Verification items for the finished model (mm, model axes). A direction names the side the tool comes from. Give positions to 0.01 mm unless a question says otherwise; leave off trailing zeros. Write each loop counter-clockwise with the first axis right and the second up, starting at its lowest first coordinate (ties: lowest second). Pieces come first, ordered by that corner, then holes. Notation, with made-up numbers: (69, -7) -> (93, -7) arc R21 ccw to (93, 5) -> close; hole circle Ø10 at (-31.5, -8.75). An arc over 180 degrees is marked (long way). Write item = value, one per line.
Autodesk Inventor part; units mm, degrees
ref_plane "YZ Plane" through (0, 0, 0) normal (1, 0, 0) x (0, 1, 0)
ref_plane "XZ Plane" through (0, 0, 0) normal (0, 1, 0) x (-1, 0, 0)
ref_plane "XY Plane" through (0, 0, 0) normal (0, 0, 1) x (1, 0, 0)
sketch "Sketch1" plane through (0, 0, 0) normal (0, 1, 0) x (-1, 0, 0)
  line L0 (0, 0) -> (100, 0)
  line L1 (100, 0) -> (100, -178)
  line L2 (0, -178) -> (0, 0)
  line L3 (90, -10) -> (10, -10)
  line L4 (90, -52) -> (10, -52)
  line L5 (90, -62) -> (10, -62)
  line L6 (90, -52) -> (90, -10)
  line L7 (10, -10) -> (10, -52)
  line L8 (90, -118) -> (10, -118)
  line L9 (90, -168) -> (90, -128)
  line L10 (90, -118) -> (90, -62)
  line L11 (10, -62) -> (10, -118)
  line L12 (10, -128) -> (10, -168)
  line L13 (100, -178) -> (90, -178)
  line L14 (10, -178) -> (0, -178)
  line L15 (90, -168) -> (90, -178)
  line L16 (10, -168) -> (46, -168)
  line L17 (56, -168) -> (56, -178)
  line L18 (56, -178) -> (10, -178)
  line L19 (56, -168) -> (56, -128)
  line L20 (46, -128) -> (46, -168)
  line L21 (90, -128) -> (56, -128)
  line L22 (46, -128) -> (10, -128)
  dimension "thickness" = 10
  dimension "d3" = 10
  dimension "d4" = 10
  dimension "d8" = 10
  dimension "motor" = 42
  dimension "d10" = 10
  dimension "d11" = 10
  dimension "d27" = 10
  dimension "batterywidth" = 56
  dimension "d31" = 80
  dimension "suspensionWidth" = 40
  dimension "d33" = 10
  dimension "d34" = 10
  dimension "suspensionHeight" = 34
  dimension "d36" = 10
  dimension "d38" = 10
  dimension "d39" = 40
  dimension "d40" = 40
  dimension "d41" = 36
extrude "Extrusion2" add sketch "Sketch1" along normal blind 10
sketch "Sketch2" plane through (0, 10, 0) normal (0, 1, 0) x (1, 0, 0)
  line L0 (-100, 0) -> (-90, 0)
  line L1 (-90, 0) -> (-90, 10)
  line L2 (-90, 10) -> (-100, 10)
  line L3 (-100, 10) -> (-100, 0)
  line L4 (-10, 52) -> (-10, 10)
  line L5 (0, 0) -> (-10, 0)
  line L6 (-10, 0) -> (-10, 10)
  line L7 (-10, 10) -> (0, 10)
  line L8 (0, 10) -> (0, 0)
  line L9 (-100, 178) -> (-100, 0)
  line L10 (-100, 0) -> (0, 0)
  line L11 (-100, 52) -> (-90, 52)
  line L12 (-90, 52) -> (-90, 62)
  line L13 (-90, 62) -> (-100, 62)
  line L14 (-100, 62) -> (-100, 52)
  line L15 (-90, 52) -> (-10, 52)
  line L16 (-10, 52) -> (0, 52)
  line L17 (0, 52) -> (0, 62)
  line L18 (0, 62) -> (-10, 62)
  line L19 (-10, 62) -> (-10, 52)
  line L20 (-90, 10) -> (-90, 52)
  line L21 (-100, 118) -> (-90, 118)
  line L22 (-90, 118) -> (-90, 128)
  line L23 (-90, 128) -> (-100, 128)
  line L24 (-100, 128) -> (-100, 118)
  line L25 (-56, 128) -> (-90, 128)
  line L26 (-56, 118) -> (-46, 118)
  line L27 (-46, 118) -> (-46, 128)
  line L28 (-46, 128) -> (-56, 128)
  line L29 (-56, 128) -> (-56, 118)
  line L30 (-90, 118) -> (-10, 118)
  line L31 (0, 178) -> (-56, 178)
  line L32 (-10, 168) -> (0, 168)
  line L33 (0, 168) -> (0, 178)
  line L34 (0, 178) -> (-10, 178)
  line L35 (-10, 178) -> (-10, 168)
  line L36 (0, 0) -> (0, 178)
  line L37 (-10, 118) -> (0, 118)
  line L38 (0, 118) -> (0, 128)
  line L39 (0, 128) -> (-10, 128)
  line L40 (-10, 128) -> (-10, 118)
  line L41 (-10, 128) -> (-46, 128)
  line L42 (-56, 158) -> (-46, 158)
  line L43 (-46, 158) -> (-46, 168)
  line L44 (-46, 168) -> (-56, 168)
  line L45 (-56, 168) -> (-56, 158)
  line L46 (-46, 168) -> (-10, 168)
  line L47 (-46, 128) -> (-46, 168)
  line L48 (-100, 158) -> (-90, 158)
  line L49 (-90, 158) -> (-90, 168)
  line L50 (-90, 168) -> (-100, 168)
  line L51 (-100, 168) -> (-100, 158)
  line L52 (-90, 128) -> (-90, 178)
  dimension "d36" = 10
  dimension "d44" = 10
  dimension "d45" = 10
  dimension "d47" = 10
  dimension "d50" = 10
  dimension "d51" = 10
  dimension "d52" = 10
  dimension "d53" = 10
  dimension "d58" = 10
  dimension "d64" = 10
  dimension "d65" = 10
  dimension "d148" = 10
  dimension "d149" = 10
  dimension "d150" = 10
  dimension "d151" = 10
extrude "Extrusion3" add sketch "Sketch2" along normal blind 10 contours L3 L2 L1 L0 | L6 L7 L8 L5 | L9 L13 L12 L11 | L19 L18 L17 L16 | L9 L23 L22 L21 | L9 L50 L49 L48 | L29 L28 L27 L26 | L37 L40 L39 L36 | L32 L35 L31 L33 | L42 L45 L44 L43
sketch "Sketch6" plane through (0, 0, 0) normal (0, -1, 0) x (1, 0, 0)
  line L0 (-90, -10) -> (-80, -10)
  line L1 (-80, -10) -> (-80, -52)
  line L2 (-80, -52) -> (-90, -52)
  line L3 (-90, -52) -> (-90, -10)
  line L4 (-90, -52) -> (-90, -10)
  line L5 (-90, -10) -> (-10, -10)
  line L6 (-10, -52) -> (-90, -52)
  line L7 (-20, -10) -> (-10, -10)
  line L8 (-10, -10) -> (-10, -52)
  line L9 (-10, -52) -> (-20, -52)
  line L10 (-20, -52) -> (-20, -10)
  line L11 (-10, -10) -> (-10, -52)
  point P0 (0, 0)
  dimension "motorFixtureHeight" = 60
  dimension "d72" = 10
extrude "Extrusion5" add sketch "Sketch6" against normal blind 10 contours L0 L1 L2 L3 | L5 L8 L6 L10
sketch "Sketch7" plane through (0, 10, 0) normal (0, 1, 0) x (1, 0, 0)
  line L0 (-80, 10) -> (-20, 10)
  line L1 (-20, 10) -> (-20, 52)
  line L2 (-20, 52) -> (-80, 52)
  line L3 (-80, 52) -> (-80, 10)
  line L4 (-80, 10) -> (-80, 52)
  line L5 (-80, 52) -> (-20, 52)
  line L6 (-20, 52) -> (-20, 10)
  line L7 (-20, 10) -> (-80, 10)
  circle A0 centre (-50, 31) radius 18.75
  circle A1 centre (-75, 16) radius 2.1
  circle A2 centre (-25, 31) radius 2.1
  circle A3 centre (-75, 46) radius 2.1
  circle A4 centre (-25, 16) radius 2.1
  circle A5 centre (-25, 46) radius 2.1
  circle A6 centre (-75, 31) radius 2.1
  point P0 (0, 0)
  dimension "d75" = 37.5
  dimension "d77" = 21
  dimension "d78" = 30
  dimension "d79" = 4.2
  dimension "d80" = 4.2
  dimension "d82" = 4.2
  dimension "d83" = 4.2
  dimension "d84" = 4.2
  dimension "d85" = 4.2
  dimension "d86" = 25
  dimension "d87" = 0
  dimension "d88" = 25
  dimension "d89" = 15
  dimension "d90" = 25
  dimension "d91" = 15
  dimension "d92" = 15
  dimension "d93" = 25
  dimension "d94" = 25
  dimension "d95" = 0
  dimension "d96" = 25
  dimension "d97" = 15
extrude "Extrusion6" add sketch "Sketch7" against normal blind 6
hole "Hole2" at (0, 15, -173) direction (-1, 0, 0) diameter 4.3 end through all
hole "Hole3" at (0, 15, -123) direction (-1, 0, 0) diameter 4.3 end through all
hole "Hole4" at (0, 15, -57) direction (-1, 0, 0) diameter 4.3 end through all
hole "Hole5" at (0, 15, -5) direction (-1, 0, 0) diameter 4.3 end through all
sketch "Sketch8" plane through (-100, 0, -178) normal (-1, 0, 0) x (0, 0, 1)
  line L0 (116, 10) -> (60, 10)
  line L1 (60, 10) -> (60, 7)
  line L2 (60, 7) -> (116, 7)
  line L3 (116, 7) -> (116, 10)
  line L4 (116, 10) -> (60, 7) construction
  line L5 (60, 10) -> (116, 7) construction
  line L6 (60, 10) -> (116, 10)
  line L7 (60, 10) -> (60, 20)
  line L8 (116, 10) -> (116, 20)
  point P0 (178, 0)
  point P1 (88, 8.5)
  dimension "d145" = 3
extrude "Extrusion7" cut sketch "Sketch8" against normal up to surface (100 mm away)
hole "Hole6" at (-95, 15, -168) direction (0, 0, 1) diameter 4.3 depth 10 tip angle 118
hole "Hole7" at (-51, 15, -168) direction (0, 0, 1) diameter 4.3 depth 10 tip angle 118
sketch "Sketch9" plane through (-56, 0, -128) normal (0, 0, -1) x (-1, 0, 0)
  circle A0 centre (27, 5) radius 3.1
  circle A1 centre (7, 5) radius 3.1
  line L0 (34, 0) -> (0, 0)
  line L1 (0, 0) -> (0, 10)
  line L2 (34, 0) -> (34, 10)
  point P0 (-56, 0)
  dimension "d170" = 6.2
  dimension "d171" = 6.2
  dimension "d172" = 5
  dimension "d173" = 5
  dimension "d174" = 7
  dimension "d175" = 7
extrude "Extrusion8" cut sketch "Sketch9" against normal blind 5
equation "\"d3\" = thickness"
equation "\"d4\" = thickness"
equation "\"d8\" = thickness"
equation "\"d10\" = thickness"
equation "\"d11\" = thickness"
equation "\"d27\" = thickness"
equation "\"d33\" = thickness"
equation "\"d34\" = thickness"
equation "\"d36\" = thickness"
equation "\"d38\" = thickness"
equation "\"d39\" = suspensionWidth"
equation "\"d40\" = suspensionWidth"
equation "\"d42\" = thickness"
equation "\"d44\" = thickness"
equation "\"d50\" = thickness"
equation "\"d51\" = thickness"
equation "\"d52\" = thickness"
equation "\"d53\" = thickness"
equation "\"d58\" = thickness"
equation "\"d64\" = thickness"
equation "\"d65\" = thickness"
equation "\"d148\" = thickness"
equation "\"d149\" = thickness"
equation "\"d150\" = thickness"
equation "\"d151\" = thickness"
equation "\"d66\" = thickness"
equation "\"d73\" = thickness"
equation "\"d77\" = 0.5 * motor"
equation "\"d159\" = thickness"
equation "\"d168\" = thickness"
properties part number "sideFrame" material "ABS Plastic"
Item 1: Sectioned sample at B-B on z = -31. Record the cut outline in (x, y), then the cut area to 3 significant figures.
Response values:
outline = (-100, 0) -> (-80, 0) -> (-80, 4) -> (-77.1, 4) -> (-77.1, 10) -> (-100, 10) -> close; (-72.9, 4) -> (-68.75, 4) -> (-68.75, 10) -> (-72.9, 10) -> close; (-31.25, 4) -> (-27.1, 4) -> (-27.1, 10) -> (-31.25, 10) -> close; (-22.9, 4) -> (-20, 4) -> (-20, 0) -> (0, 0) -> (0, 10) -> (-22.9, 10) -> close
area = 485 mm^2
Item 2: Go/stop test with flat-tipped pins: P1, Ø8, axis at x = -96, z = -76.5, coming from the +Y side; P2, Ø4, axis at x = -66, z = -118.5, coming from the +Y side; P3, Ø4, axis at y = 15, z = -173, coming from the +X side; P4, Ø3, axis at x = -82, y = 5, coming from the -Z side. Record where each tip stops, or that it passes through.
Response values:
P1 = 7
P2 = 10
P3 = through
P4 = -123
Item 3: Sectioned sample at C-C on x = -51. Record the cut outline in (y, z).
Response values:
outline = (0, -178) -> (10, -178) -> (10, -168) -> (12.85, -168) -> (12.85, -158) -> (10, -158) -> (10, -128) -> (20, -128) -> (20, -118) -> (0, -118) -> close; (0, -62) -> (10, -62) -> (10, -49.72) -> (4, -49.72) -> (4, -52) -> (0, -52) -> close; (0, -10) -> (4, -10) -> (4, -12.28) -> (10, -12.28) -> (10, 0) -> (0, 0) -> close; (17.15, -168) -> (20, -168) -> (20, -158) -> (17.15, -158) -> close; hole circle Ø4.3 at (15, -123)
Item 4: Set-up check for faces 1 (the cylindrical face through (-52.81, 16.16, -162.93)), 2 (the flat face through (-46, 8, -152)), 3 (the flat face through (-90, 12.7, -4.9)), 4 (the flat face through (-51, 10, -143)): record each of +Z, -Z, +X, -X, +Y, -Y from which the full face is reachable in a straight line by a thin tool's end or side.
Response values:
face_1 = -Z
face_2 = +Y, -Y
face_3 = +Z, -Z, +Y
face_4 = +X, -X, +Y
Item 5: Mould release check, pull along X, two halves, no side actions. Record for faces 5 (the flat face through (-10, 14.9, -175.3)), 6 (the flat face through (-28, 10, -123)), 7 (the flat face through (-5, 20, -173)): +X half, -X half, draft (parallel to the pull), parting line (faces both ways), or undercut.
Response values:
face_5 = -X half
face_6 = undercut
face_7 = draft
Item 6: Material ranges on line 1 (X direction, y = 5.35, z = -31); line 2 (Z direction, x = -75, y = 6.5); line 3 (X direction, y = 9, z = -155), recorded low to high.
Response values:
line_1 = -100 to -77.1, -72.9 to -68.75, -31.25 to -27.1, -22.9 to 0
line_2 = -128 to -118, -62 to -48.1, -43.9 to -33.1, -28.9 to -18.1, -13.9 to 0
line_3 = -100 to -90, -56 to -46, -10 to 0
Item 7: Sectioned sample at A-A on x = -95. Record the cut outline in (y, z), then the cut area to 3 significant figures.
Response values:
outline = (0, -178) -> (10, -178) -> (10, -168) -> (12.85, -168) -> (12.85, -158) -> (10, -158) -> (10, -128) -> (20, -128) -> (20, -118) -> (7, -118) -> (7, -62) -> (20, -62) -> (20, -52) -> (10, -52) -> (10, -10) -> (20, -10) -> (20, 0) -> (0, 0) -> close; (17.15, -168) -> (20, -168) -> (20, -158) -> (17.15, -158) -> close; hole circle Ø4.3 at (15, -123); hole circle Ø4.3 at (15, -57); hole circle Ø4.3 at (15, -5)
area = 1,930 mm^2
Item 8: Sectioned sample at D-D on z = -5. Record the cut outline in (x, y), then the cut area to 3 significant figures.
Response values:
outline = (-100, 0) -> (0, 0) -> (0, 12.85) -> (-10, 12.85) -> (-10, 10) -> (-90, 10) -> (-90, 12.85) -> (-100, 12.85) -> close; (-100, 17.15) -> (-90, 17.15) -> (-90, 20) -> (-100, 20) -> close; (-10, 17.15) -> (0, 17.15) -> (0, 20) -> (-10, 20) -> close
area = 1,110 mm^2
